Verification items for this drawing (mm, ordinates from the low corner). Round coordinates to 2 decimals unless told otherwise and drop trailing zeros. Loops run counter-clockwise (first coordinate to the right, second up) from the corner with the lowest first, then second, coordinate; pieces in that order, holes last. Notation, with made-up numbers: (-23.75, 64) - (-1.75, 64) arc R13 cw to (-1.75, 71) - close; hole circle Ø2 at (-7, 74.25). An arc over 180 degrees is marked (long way). Write item = value, one per line.
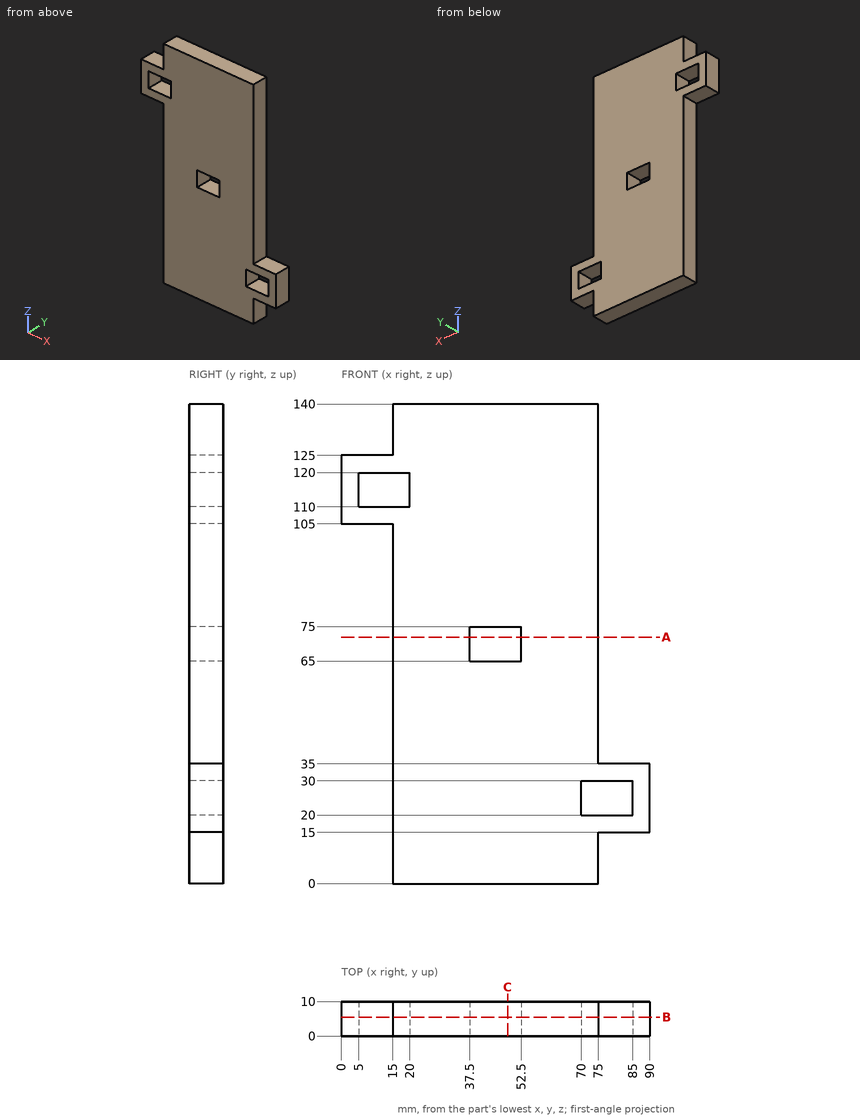
(1) Section check A-A (z = 72). Enter the section's corners in (x, y).
Answers follow:
outline = (15, 0) - (37.5, 0) - (37.5, 10) - (15, 10) - close; (52.5, 0) - (75, 0) - (75, 10) - (52.5, 10) - close
(2) Section check C-C (x = 48.5). Enter the section's corners in (y, z).
Answers follow:
outline = (0, 0) - (10, 0) - (10, 65) - (0, 65) - close; (0, 75) - (10, 75) - (10, 140) - (0, 140) - close
(3) Gauge pin test, flat ends, axial feed: pin 1 (5 mm diameter, centred on y = 4.5, z = 72.5, fed in from -X); pin 2 (3 mm diameter, centred on y = 6, z = 110.5, fed in from +X); pin 3 (3 mm diameter, centred on x = 78, y = 4, fed in from -Z). Record the tip position at first contact, or that the pin passes through.
Answers follow:
pin_1 = 15
pin_2 = 75
pin_3 = 15
(4) Section check B-B (y = 5.5). Enter the section's corners in (x, z), then the cut area to 3 significant figures.
Answers follow:
outline = (0, 105) - (15, 105) - (15, 0) - (75, 0) - (75, 15) - (90, 15) - (90, 35) - (75, 35) - (75, 140) - (15, 140) - (15, 125) - (0, 125) - close; hole (5, 110) - (20, 110) - (20, 120) - (5, 120) - close; hole (37.5, 65) - (52.5, 65) - (52.5, 75) - (37.5, 75) - close; hole (70, 20) - (85, 20) - (85, 30) - (70, 30) - close
area = 8,550 mm²
(5) Scan lines: L1, parallel to Z at x = 49, y = 3.25; L2, parallel to X at y = 9, z = 25.5; L3, parallel to Z at x = 14.5, y = 1. Record each from-to range of solid material in increasing order. Write a range as [from, to].
Answers follow:
L1 = [0, 65], [75, 140]
L2 = [15, 70], [85, 90]
L3 = [105, 110], [120, 125]
